Geometry: see drawing. Coordinates: mm, zero at the bounding-box minimum. Round coordinates to 2 decimals unless told otherwise and drop trailing zeros. Write each loop counter-clockwise with the first axis right and the second up, starting at its lowest first coordinate (ties: lowest second). Pieces come first, ordered by that corner, then holes. Notation, with made-up numbers: M -39,82.5 L -18,82.5 A22 cw -18,107.5 Z; hole C 63,24.5 d2. An arc over 180 degrees is marked long. Use one line per item in the form item = value. Start each with the question number.
Item 1: Section query A-A (z = 155). Return loops of the section in (x, y), and give its area (3 significant figures).
Item 2: Section query C-C (y = 3.75). Return loops of the section in (x, z).
Item 3: Section query B-B (x = 9.25). Return loops of the section in (y, z).
Item 4: Ray query, probe 1 along X at (y, z) = (0.7, 77); probe 2 along Z at (x, y) = (4.75, 0.8); probe 3 along Z at (x, y) = (15.25, 2.4). Return the intervals inside material, ascending.
Item 5: Pin query (flat end, axial travel): pin 1 Ø5 at (x, z) = (8.5, 196.5) entering from +Y. Return the tip coordinate at first contact, or that it passes through.
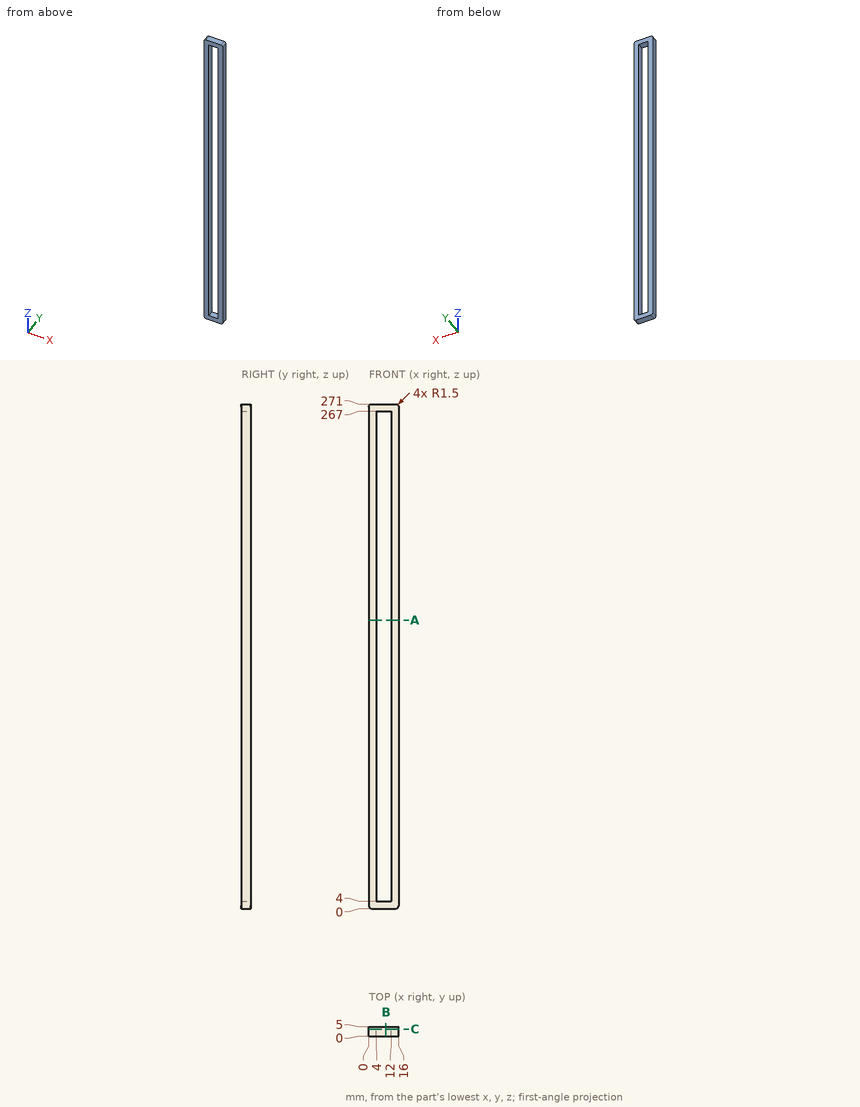
Working result:
q1.outline = M 0,0 L 4,0 L 4,5 L 0,5 Z; M 12,0 L 16,0 L 16,5 L 12,5 Z
q1.area = 40.0 mm²
q2.outline = M 0,1.5 A1.5 ccw 1.5,0 L 14.5,0 A1.5 ccw 16,1.5 L 16,269.5 A1.5 ccw 14.5,271 L 1.5,271 A1.5 ccw 0,269.5 Z; hole M 4,4 L 12,4 L 12,267 L 4,267 Z
q3.outline = M 0,0 L 5,0 L 5,4 L 0,4 Z; M 0,267 L 5,267 L 5,271 L 0,271 Z
q4.probe_1 = 0 to 4, 12 to 16
q4.probe_2 = 0 to 4, 267 to 271
q4.probe_3 = 0.2 to 270.8
q5.pin_1 = through
